Design review of the part built by this model. Coordinates are the model's own, in mm. A direction names the side the tool comes from. Coordinates: 2 decimals unless noted, no trailing zeros. Order: outer loops, then holes, each group sorted by start corner. A loop starts at its lowest first (then second) coordinate and runs counter-clockwise, first axis right, second up. Notation, with made-up numbers: (19, 25.5) -> (65, 25.5) arc R27 ccw to (65, 60.5) -> close; hole circle Ø3 at (67.25, 11). An arc over 180 degrees is marked (long way). Use a Markdown table: item, result. Add a question column.
Q1. Machinability: for faces 5 (the face through (0, 22, 6)), 6 (the face through (17, 22, 8.5)), which of the approach directions +Z, -Z, +X, -X, +Y, -Y give a long, thin tool a straight path to every point of the face, cutting with its end or side? Answer none if there is none.
Q2. The part is to be moulded in two halves that separate along Z. For faces 1 (the face through (18, 22, 3.5)), 2 (the face through (49, 23, 0)), 3 (the face through (49, 23, 12)), 4 (the face through (49, 45, 6)), say which applies: pulls with the +Z half, pulls with the -Z half, needs draft (parallel to the pull), parting line crosses it, or undercut.
Q3. Add section C-C (z = 6). State the section outline as (x, y) points, then the cut area to 4 significant figures.
Q4. Wall thickness on probe 1 along X at (y, z) = (16.5, 6); probe 2 along Z at (x, y) = (19.5, 20); probe 3 along X at (y, z) = (11, 3.75): over which ranges is each line inside the solid? List them lowest first.
Q5. Add section A-A (x = 95). State the section outline as (y, z) points.
Q6. Add section B-B (y = 15.5). State the section outline as (x, z) points.
Q7. Insertion check: pin 1 (6 mm diameter, centred on x = 29.5, z = 7, fed in from -Y). The pin has a flat end and moves straight along its axis. Give the tip position at first contact, or say it passes through.
from build123d import *

# Parameters (mm, degrees)
SKETCH3_W           = 100
SKETCH3_H           = 45
BOSS_EXTRUDE2_DEPTH = 12
SKETCH4_R           = 2.5
CUT_EXTRUDE1_DEPTH  = 111.313190508


with BuildPart() as part:
    # Sketch3 → Boss-Extrude2 (new body)
    with BuildSketch(Plane.XY):
        with Locations((50, 22.5)):
            Rectangle(SKETCH3_W, SKETCH3_H)
    extrude(amount=BOSS_EXTRUDE2_DEPTH)

    # Sketch4 → Cut-Extrude1 (cut, through all)
    with BuildSketch(Plane.XZ):
        with Locations(Location((95, 6, 0), (0, 0, 270))):
            Circle(SKETCH4_R)
        with BuildLine():
            Line((30, 3.5), (5, 3.5))
            ThreePointArc((5, 3.5), (2.5, 6), (5, 8.5))
            Line((5, 8.5), (30, 8.5))
            ThreePointArc((30, 8.5), (32.5, 6), (30, 3.5))
        make_face()
    extrude(amount=-CUT_EXTRUDE1_DEPTH, mode=Mode.SUBTRACT)


solid = part.part
Established:
| question | item | result |
|---|---|---|
| 1 | face 5 | +Z, -Z, -X, +Y, -Y |
| 1 | face 6 | +Y, -Y |
| 2 | face 1 | undercut |
| 2 | face 2 | pulls with the -Z half |
| 2 | face 3 | pulls with the +Z half |
| 2 | face 4 | needs draft |
| 3 | outline | (0, 0) -> (2.5, 0) -> (2.5, 45) -> (0, 45) -> close; (32.5, 0) -> (92.5, 0) -> (92.5, 45) -> (32.5, 45) -> close; (97.5, 0) -> (100, 0) -> (100, 45) -> (97.5, 45) -> close |
| 3 | area | 2,925 mm^2 |
| 4 | probe 1 | 0 to 2.5, 32.5 to 92.5, 97.5 to 100 |
| 4 | probe 2 | 0 to 3.5, 8.5 to 12 |
| 4 | probe 3 | 0 to 3.91, 31.09 to 93.91, 96.09 to 100 |
| 5 | outline | (0, 0) -> (45, 0) -> (45, 3.5) -> (0, 3.5) -> close; (0, 8.5) -> (45, 8.5) -> (45, 12) -> (0, 12) -> close |
| 6 | outline | (0, 0) -> (100, 0) -> (100, 12) -> (0, 12) -> close; hole (5, 3.5) -> (30, 3.5) arc R2.5 ccw to (30, 8.5) -> (5, 8.5) arc R2.5 ccw to start; hole circle Ø5 at (95, 6) |
| 7 | pin 1 | y = 0 |
